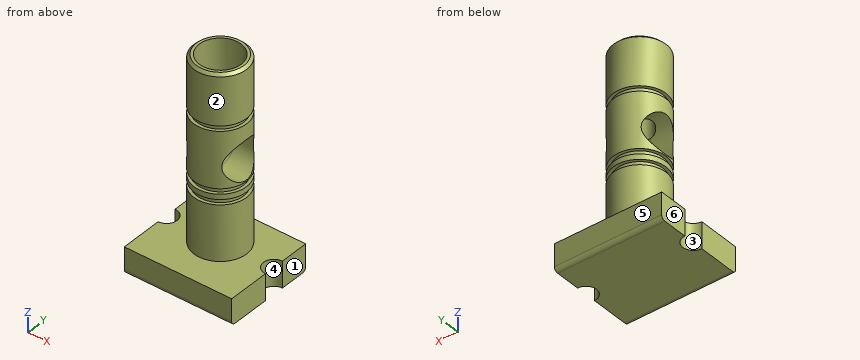
from build123d import *

# Parameters (mm, degrees)
BOSS_EXTRUDE1_DEPTH     = 20
SKETCH2_R               = 20
BOSS_EXTRUDE2_DEPTH     = 139
SKETCH3_R               = 15
CUT_EXTRUDE1_DEPTH      = 42
CUT_EXTRUDE1_DEPTH_BACK = 42
SKETCH4_W               = 4
SKETCH4_H               = 2.3
SKETCH5_R               = 16
CUT_EXTRUDE2_DEPTH      = 35.4
SKETCH6_R               = 9.5
CUT_EXTRUDE3_DEPTH      = 22
CHAMFER1_SIZE           = 2
FILLET1_R               = 3


with BuildPart() as part:
    # Sketch1 → Boss-Extrude1 (new body)
    with BuildSketch(Plane.XY):
        with BuildLine():
            Line((-41, -8), (-41, -40))
            Line((-41, -40), (41, -40))
            Line((41, -40), (41, -8))
            ThreePointArc((41, -8), (33, 0), (41, 8))
            Line((41, 8), (41, 30))
            Line((41, 30), (-41, 30))
            Line((-41, 30), (-41, 8))
            ThreePointArc((-41, 8), (-33, 0), (-41, -8))
        make_face()
    extrude(amount=BOSS_EXTRUDE1_DEPTH)

    # Sketch2 → Boss-Extrude2 (add)
    with BuildSketch(Plane.XY.offset(20)):
        Circle(SKETCH2_R)
    extrude(amount=BOSS_EXTRUDE2_DEPTH)

    # Sketch3 → Cut-Extrude1 (cut, two sides)
    with BuildSketch(Plane(origin=(0, 0, 0), x_dir=(0, 0, -1), z_dir=(1, 0, 0))) as cut_extrude1_sk:
        with Locations((-90, 0)):
            Circle(SKETCH3_R)
    extrude(amount=CUT_EXTRUDE1_DEPTH, mode=Mode.SUBTRACT)
    extrude(cut_extrude1_sk.sketch, amount=-CUT_EXTRUDE1_DEPTH_BACK, mode=Mode.SUBTRACT)

    # Sketch4 → Cut-Revolve1 (revolve, cut)
    with BuildSketch(Plane(origin=(0, 0, 0), x_dir=(0, 0, -1), z_dir=(1, 0, 0))):
        with Locations((-64, 18.85)):
            Rectangle(SKETCH4_W, SKETCH4_H)
        with Locations((-72, 18.85)):
            Rectangle(SKETCH4_W, SKETCH4_H)
        with Locations((-118.6, 18.85)):
            Rectangle(SKETCH4_W, SKETCH4_H)
    revolve(axis=Axis((0, 0, 0), (0, 0, 1)), mode=Mode.SUBTRACT)

    # Sketch5 → Cut-Extrude2 (cut)
    with BuildSketch(Plane.XY.offset(159)):
        Circle(SKETCH5_R)
    extrude(amount=-CUT_EXTRUDE2_DEPTH, mode=Mode.SUBTRACT)

    # Sketch6 → Cut-Extrude3 (cut)
    with BuildSketch(Plane.XY.offset(123.6)):
        Circle(SKETCH6_R)
    extrude(amount=-CUT_EXTRUDE3_DEPTH, mode=Mode.SUBTRACT)

    # Chamfer1
    chamfer1_edges = [part.edges().sort_by_distance(p)[0] for p in [
        (-20, 0, 159),
    ]]
    chamfer(chamfer1_edges, length=CHAMFER1_SIZE)

    # Fillet1
    fillet1_edges = [part.edges().sort_by_distance(p)[0] for p in [
        (0, -40, 0),
        (0, 30, 0),
    ]]
    fillet(fillet1_edges, radius=FILLET1_R)


solid = part.part
Geometry: final body of the model. Coordinates: model frame, mm. Face numbers are marked on the shaded views. A direction names the side the tool comes from. Give positions to 0.01 mm unless a question says otherwise; leave off trailing zeros. Loops run counter-clockwise (first coordinate to the right, second up) from the corner with the lowest first, then second, coordinate; pieces in that order, holes last. Notation, with made-up numbers: (76.5, -33.75) - (84.5, -33.75) arc R26 ccw to (84.5, -8.75) - close; hole circle Ø11 at (74, 10.5). An arc over 180 degrees is marked (long way). One line per question, with ' | ' between items. Start each with the question number.
(1) Section query B-B on y = 0. Count the separate pieces of the cut face and the enclosed holes in it, then the cut area to 3 significant figures.
(2) Reachability of the marked faces 1 and 2 from +Z, -Z, +X, -X, +Y, -Y: full face, straight path, thin tool, end or side. Return the list, or none.
(3) Ray query, line 1 (Y direction, x = 0, z = 135); line 2 (X direction, y = 0, z = 108); line 3 (Z direction, x = -31, y = -31.5). Return the intervals inside material, ascending. Write a range as from..to.
(4) Contact query for flat-ended pins moving along their axis: pin 1 (6 mm diameter, centred on x = 1.5, z = 65.5, fed in from -Y); pin 2 (8 mm diameter, centred on x = 26, y = -0.5, fed in from +Z); pin 3 (1.5 mm diameter, centred on x = 22.5, z = 57, fed in from -Y); pin 4 (12 mm diameter, centred on x = -7, y = 5, fed in from +Z). Output: stop coordinate, or through.
(5) Pull-direction query (Y, two-part tool) for the marked faces 3, 4, 5 and 6; classes: released by +Y, released by -Y, zero draft, split by the parting line, or undercut.
(6) Section query C-C on z = 89. Return loops of the section in (x, y), then the cut area to 3 significant figures.
(7) Section query D-D on y = -23.5. Return loops of the section in (x, z).
(8) Section query A-A on x = 24. Return loops of the section in (y, z), then the cut area to 3 significant figures.
The answers:
1) separate pieces: 3 | enclosed holes: 0 | area: 4,130 mm2
2) face 1: +Z, -Z, +X, +Y, -Y | face 2: +Z
3) line 1: -20..-16, 16..20 | line 2: -20..-9.5, 9.5..20 | line 3: 0..20
4) pin 1: y = -20 | pin 2: z = 20 | pin 3: through | pin 4: z = 123.6
5) face 3: undercut | face 4: undercut | face 5: released by +Y | face 6: zero draft
6) outline: (-13.27, -14.97) arc R20 ccw to (13.27, -14.97) - close; (-13.27, 14.97) - (13.27, 14.97) arc R20 ccw to start | area: 183 mm2
7) outline: (-41, 0) - (41, 0) - (41, 20) - (-41, 20) - close
8) outline: (-40, 3) arc R3 ccw to (-37, 0) - (27, 0) arc R3 ccw to (30, 3) - (30, 20) - (-40, 20) - close | area: 1,400 mm2
